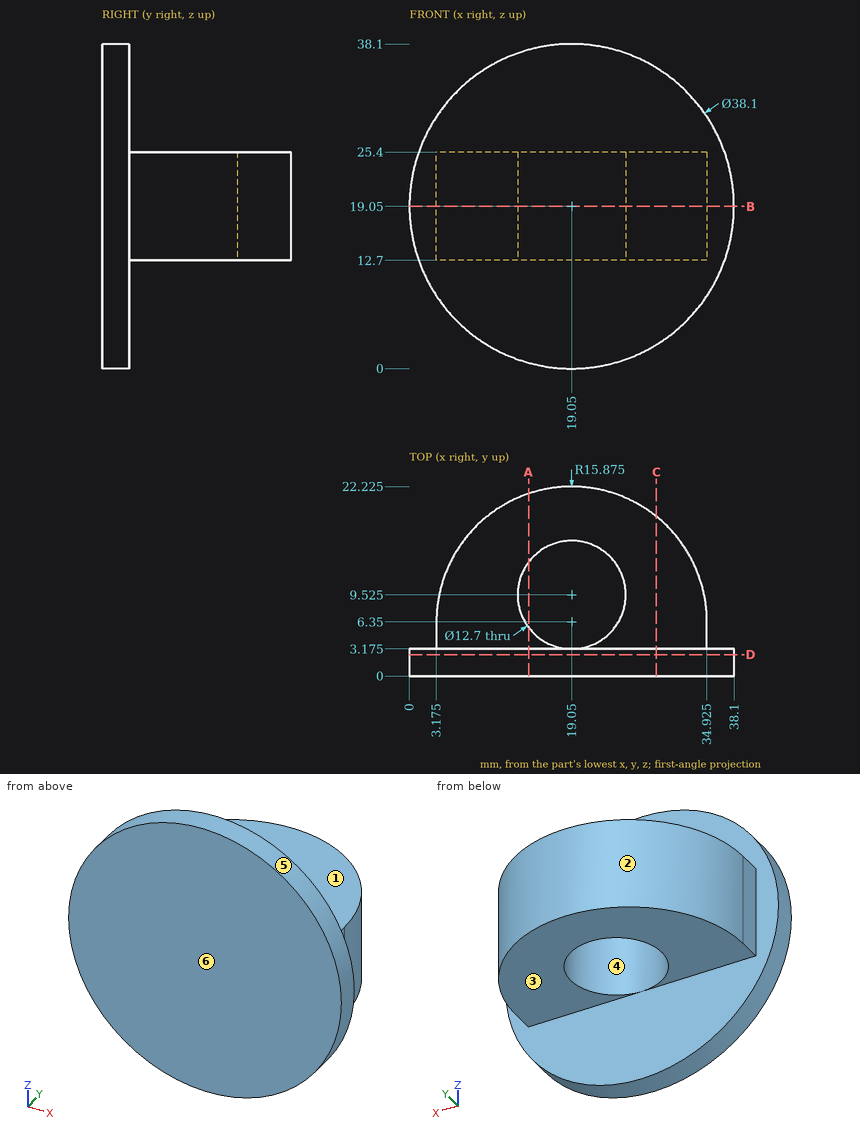
The drawing under review shows one solid part. Ordinate dimensions are in mm from its lowest x, y, z. A direction names the side the tool comes from. Round coordinates to 2 decimals unless told otherwise and drop trailing zeros. Loops run counter-clockwise (first coordinate to the right, second up) from the corner with the lowest first, then second, coordinate; pieces in that order, holes last. Notation, with made-up numbers: (36.5, -20.75) -> (80.5, -20.75) arc R29 ccw to (80.5, 13.25) -> close; hole circle Ø3 at (50.25, 1.5). An arc over 180 degrees is marked (long way). Answer in a Markdown table with one row per item.
1) Consider section A-A, the plane x = 14. Write out the cut boundary in (y, z) (3 decimals).
Taken from the geometry:
| item | result |
|---|---|
| outline | (0, 0.682) -> (3.175, 0.682) -> (3.175, 12.7) -> (5.675, 12.7) -> (5.675, 25.4) -> (3.175, 25.4) -> (3.175, 37.418) -> (0, 37.418) -> close; (13.375, 12.7) -> (21.4, 12.7) -> (21.4, 25.4) -> (13.375, 25.4) -> close |
2) Draft analysis for pull direction X (two halves, no side actions). For the marked faces 4, 5 and 6, state which applies: pulls with the +X half, pulls with the -X half, needs draft (parallel to the pull), parting line crosses it, or undercut.
Taken from the geometry:
| item | result |
|---|---|
| face 4 | undercut |
| face 5 | parting line crosses it |
| face 6 | needs draft |
3) Tool access review of the marked faces 1, 2 and 3: name each direction out of +Z, -Z, +X, -X, +Y, -Y from which nothing blocks a thin tool from reaching the whole face with its end or side.
Taken from the geometry:
| item | result |
|---|---|
| face 1 | +Z, +X, -X, +Y |
| face 2 | +Z, -Z, +Y |
| face 3 | -Z, +X, -X, +Y |
4) Wall thickness on line 1 along Y through (x, z) = (19.05, 20.75) (3 decimals); line 2 along Z through (x, y) = (6.5, 11.25); line 3 along Y through (x, z) = (4, 30) (3 decimals): over which ranges is each line inside the solid? List them lowest first.
Taken from the geometry:
| item | result |
|---|---|
| line 1 | y = 0 to 3.175, 15.875 to 22.225 |
| line 2 | z = 12.7 to 25.4 |
| line 3 | y = 0 to 3.175 |
5) For pin 1 Ø1 at (y, z) = (5.5, 19.5) entering from +X (3 decimals); pin 2 Ø1 at (x, y) = (23, 19.5) entering from -Z; pin 3 Ø1 at (x, z) = (8, 12.5) entering from +Y (3 decimals); pin 4 Ø11.5 at (x, z) = (20.5, 23) entering from +Y (3 decimals), all flat-tipped, find the tip position at first contact; note any pin that passes through.
Taken from the geometry:
| item | result |
|---|---|
| pin 1 | stops at x = 34.925 |
| pin 2 | stops at z = 12.7 |
| pin 3 | stops at y = 18.175 |
| pin 4 | stops at y = 22.225 |
6) Consider section C-C, the plane x = 29. Write out the cut boundary in (y, z) (3 decimals).
Taken from the geometry:
| item | result |
|---|---|
| outline | (0, 2.805) -> (3.175, 2.805) -> (3.175, 12.7) -> (18.72, 12.7) -> (18.72, 25.4) -> (3.175, 25.4) -> (3.175, 35.295) -> (0, 35.295) -> close |
7) Consider section B-B, the plane z = 19.05. Write out the cut boundary in (x, y) (3 decimals).
Taken from the geometry:
| item | result |
|---|---|
| outline | (0, 0) -> (38.1, 0) -> (38.1, 3.175) -> (34.925, 3.175) -> (34.925, 6.35) arc R15.875 ccw to (3.175, 6.35) -> (3.175, 3.175) -> (0, 3.175) -> close; hole circle Ø12.7 at (19.05, 9.525) |
8) Consider section D-D, the plane y = 2.5. Write out the cut boundary in (x, z), plus the area to 3 significant figures.
Taken from the geometry:
| item | result |
|---|---|
| outline | circle Ø38.1 at (19.05, 19.05) |
| area | 1,140 mm² |
